The model under review builds one solid part; all positions refer to its coordinate system, in mm. Round coordinates to 2 decimals unless told otherwise and drop trailing zeros. Order: outer loops, then holes, each group sorted by start corner. A loop starts at its lowest first (then second) coordinate and runs counter-clockwise, first axis right, second up. Notation, with made-up numbers: (-11, 9) - (2, 9) arc R28 ccw to (2, 40) - close; hole circle Ø9 at (22.25, 76). An arc over 180 degrees is marked (long way). One line per question, with ' | ' between items. Start each with the question number.
Item 1: Add section C-C on y = 2.5. State the section outline as (x, z) points, and give its area (3 significant figures).
Item 2: Add section B-B on z = 10.5. State the section outline as (x, y) points.
Item 3: Add section D-D on x = 11.5. State the section outline as (y, z) points.
Item 4: For L1, parallel to X at y = 0.5, z = 4.5; L2, parallel to Y at x = 13.75, z = 2.5; L3, parallel to X at y = -5.5, z = 1.5, list the stretches that pass through material, from the lowest coordinate up. Write a range as [from, to].
Item 5: Add section A-A on x = -13.75. State the section outline as (y, z) points.
Item 6: Draft analysis for pull direction Y (two halves, no side actions). For faces 1 (the face through (-27.861, 12.745, 6.084)), 2 (the face through (22.334, 2.703, 5.916)), 3 (the face through (0, 0, 12)), 4 (the face through (-5.166, 2.703, 5.916)), state which applies: +Y half, -Y half, draft (parallel to the pull), parting line (faces both ways), or undercut.
from build123d import *

# Parameters (mm, degrees)
F0_W     = 60
F0_H     = 30
F0_R     = 9
F1_DEPTH = 12
F2_R     = 7.5
F3_R     = 7.5
F4_R     = 7.5
F5_R     = 7.5


with BuildPart() as f1:
    # F0 (on Top) → F1 (new body)
    with BuildSketch(Plane.XY):
        Rectangle(F0_W, F0_H)
        with Locations((-13.75, 0)):
            Circle(F0_R, mode=Mode.SUBTRACT)
        with Locations((13.75, 0)):
            Circle(F0_R, mode=Mode.SUBTRACT)
    extrude(amount=F1_DEPTH)

    # F2
    f2_edges = [f1.edges().sort_by_distance(p)[0] for p in [
        (-30, -15, 6),
    ]]
    fillet(f2_edges, radius=F2_R)

    # F3
    f3_edges = [f1.edges().sort_by_distance(p)[0] for p in [
        (-30, 15, 6),
    ]]
    fillet(f3_edges, radius=F3_R)

    # F4
    f4_edges = [f1.edges().sort_by_distance(p)[0] for p in [
        (30, -15, 6),
    ]]
    fillet(f4_edges, radius=F4_R)

    # F5
    f5_edges = [f1.edges().sort_by_distance(p)[0] for p in [
        (30, 15, 6),
    ]]
    fillet(f5_edges, radius=F5_R)


solid = f1.part
Determined:
1) outline: (-30, 0) - (-22.4, 0) - (-22.4, 12) - (-30, 12) - close; (-5.1, 0) - (5.1, 0) - (5.1, 12) - (-5.1, 12) - close; (22.4, 0) - (30, 0) - (30, 12) - (22.4, 12) - close | area: 305 mm2
2) outline: (-30, -7.5) arc R7.5 ccw to (-22.5, -15) - (22.5, -15) arc R7.5 ccw to (30, -7.5) - (30, 7.5) arc R7.5 ccw to (22.5, 15) - (-22.5, 15) arc R7.5 ccw to (-30, 7.5) - close; hole circle Ø18 at (-13.75, 0); hole circle Ø18 at (13.75, 0)
3) outline: (-15, 0) - (-8.71, 0) - (-8.71, 12) - (-15, 12) - close; (8.71, 0) - (15, 0) - (15, 12) - (8.71, 12) - close
4) L1: [-30, -22.74], [-4.76, 4.76], [22.74, 30] | L2: [-15, -9], [9, 15] | L3: [-30, -20.87], [-6.63, 6.63], [20.87, 30]
5) outline: (-15, 0) - (-9, 0) - (-9, 12) - (-15, 12) - close; (9, 0) - (15, 0) - (15, 12) - (9, 12) - close
6) face 1: +Y half | face 2: undercut | face 3: draft | face 4: undercut
